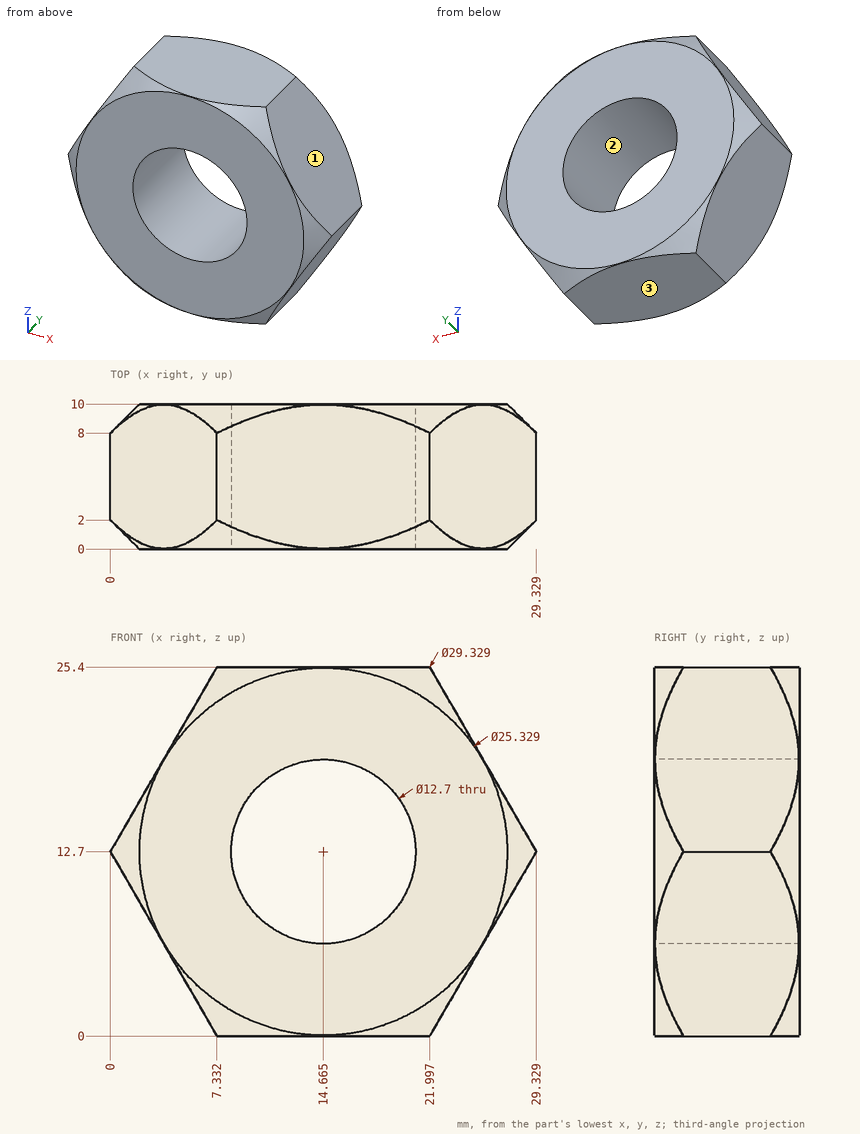
Print and shaded views of the part. All mm, measured from the part's lowest x, y and z. Coordinates: 2 decimals unless noted, no trailing zeros. One line per question, with ' | ' between items. Start each with the question number.
Q1. Pin check, flat tips, straight feed: pin 1 (5 mm diameter, centred on y = 6.5, z = 22.5, fed in from -X) (1 decimal); pin 2 (2 mm diameter, centred on y = 7.5, z = 8.5, fed in from -X). Stop position of each tip, or through.
Q2. Drill centre lines: line 1 (Z direction, x = 14.5, y = 2.5); line 2 (Z direction, x = 9, y = 5.5); line 3 (X direction, y = 3.25, z = 17.25) (1 decimal). Where is each one in solid material? Low to high. Write a range as [from, to].
Q3. Pull direction X, two halves, no side cores. Call the marked faces 1, 2 and 3: pulls with the +X half, pulls with the -X half, needs draft (parallel to the pull), parting line crosses it, or undercut.
Answer below:
1) pin 1: x = 4.2 | pin 2: x = 1.85
2) line 1: [0, 6.35], [19.05, 25.4] | line 2: [0, 9.83], [15.57, 25.4] | line 3: [2.6, 10.2], [19.1, 26.7]
3) face 1: pulls with the +X half | face 2: undercut | face 3: needs draft
